Model file for the job. Use its own axes, mm. A direction names the side the tool comes from. Round coordinates to 2 decimals unless told otherwise and drop trailing zeros. Loops run counter-clockwise (first coordinate to the right, second up) from the corner with the lowest first, then second, coordinate; pieces in that order, holes last. Notation, with made-up numbers: (47, 51) - (77, 51) arc R22 ccw to (77, 60) - close; hole circle Ø3 at (0, 86.5). An arc over 180 degrees is marked (long way). Use one line per item in the form item = value.
from build123d import *

# Parameters (mm, degrees)
SKETCH_1_R          = 7.5
SKETCH_1_R_2        = 3
EXTRUDE_1_DEPTH     = 5
SKETCH_2_R          = 7.5
SKETCH_2_R_2        = 6.5
CUT_EXTRUDE_1_DEPTH = 3.9
CHAMFER_1_SIZE      = 0.1
CHAMFER_1_SIZE2     = 0.119175359


with BuildPart() as part:
    # 草图1 → 凸台-拉伸1 (new body)
    with BuildSketch(Plane.XY):
        Circle(SKETCH_1_R)
        Circle(SKETCH_1_R_2, mode=Mode.SUBTRACT)
    extrude(amount=EXTRUDE_1_DEPTH)

    # 草图2 → 切除-拉伸1 (cut)
    with BuildSketch(Plane.XY.offset(5)):
        Circle(SKETCH_2_R)
        Circle(SKETCH_2_R_2, mode=Mode.SUBTRACT)
    extrude(amount=-CUT_EXTRUDE_1_DEPTH, mode=Mode.SUBTRACT)

    # 倒角1
    chamfer_1_edges = [part.edges().sort_by_distance(p)[0] for p in [
        (-3, 0, 0),
    ]]
    chamfer_1_side = [part.faces().sort_by_distance(p)[0] for p in [
        (-3, 0, 2.5),
    ]]
    chamfer(chamfer_1_edges, length=CHAMFER_1_SIZE, length2=CHAMFER_1_SIZE2, reference=chamfer_1_side[0])


solid = part.part
1. Wall check: probe 1 along Y at (x, z) = (0, 1.9); probe 2 along X at (y, z) = (2, 0.45); probe 3 along Z at (x, y) = (4.5, -5.25). Give the ranges that are in metal, low to high.
Geometry check:
probe_1 = -6.5 to -3, 3 to 6.5
probe_2 = -7.23 to -2.24, 2.24 to 7.23
probe_3 = 0 to 1.1
2. Cut at C-C, the plane x = -4.75. Give the cut face in (y, z), plus the area to 3 significant figures.
Geometry check:
outline = (-5.8, 0) - (5.8, 0) - (5.8, 1.1) - (4.44, 1.1) - (4.44, 5) - (-4.44, 5) - (-4.44, 1.1) - (-5.8, 1.1) - close
area = 47.4 mm^2
3. Tool access for faces 4 (the flat face through (-6, 3, 1.1)), 5 (the cylindrical face through (-7.493, 0.33, 0.542)): list every direction of +Z, -Z, +X, -X, +Y, -Y with a clear straight run to the whole face (end or side of a thin tool).
Geometry check:
face_4 = +Z
face_5 = +Z, -Z
4. Cut at D-D, the plane z = 3.45. Give the cut face in (x, y), plus the area to 3 significant figures.
Geometry check:
outline = circle Ø13 at (0, 0); hole circle Ø6 at (0, 0)
area = 104 mm^2
5. Cut at A-A, the plane y = 0. Give the cut face in (x, z).
Geometry check:
outline = (-7.5, 0) - (-3.12, 0) - (-3, 0.1) - (-3, 5) - (-6.5, 5) - (-6.5, 1.1) - (-7.5, 1.1) - close; (3, 0.1) - (3.12, 0) - (7.5, 0) - (7.5, 1.1) - (6.5, 1.1) - (6.5, 5) - (3, 5) - close
6. Pull direction X, two halves, no side cores. Call faces 1 (the flat face through (3, -1, 5)), 2 (the cylindrical face through (-3, 0, 3)), 3 (the cylindrical face through (-5.158, -3.955, 3.077)): +X half, -X half, draft (parallel to the pull), parting line (faces both ways), or undercut.
Geometry check:
face_1 = draft
face_2 = undercut
face_3 = parting line
7. Flat gauge pins, fed straight in: pin 1 (1 mm diameter, centred on y = 5, z = 3.5, fed in from +X); pin 2 (2 mm diameter, centred on x = -6, z = 3, fed in from +Y); pin 3 (1.5 mm diameter, centred on x = -4.5, z = 3.5, fed in from +Y). Where does each tip first touch, or does it go through?
Geometry check:
pin_1 = 4.69
pin_2 = 4.15
pin_3 = 5.31
